Check sheet for the modelled part. Datum: model origin and axes. Units: mm. Face numbers are marked on the shaded views. Round coordinates to 2 decimals unless told otherwise and drop trailing zeros. Write each loop counter-clockwise with the first axis right and the second up, starting at its lowest first coordinate (ties: lowest second). Pieces come first, ordered by that corner, then holes.
Item 1: Cross-section at C-C on x = 91. Enter the section's corners in (y, z).
Item 2: Cross-section at A-A on z = 7.5. Enter the section's corners in (x, y), plus the area to 3 significant figures.
Item 3: Release check for a two-part mould opening along X. For the marked faces 1 and 2 record: +X half, -X half, draft (parallel to the pull), parting line (faces both ways), or undercut.
Item 4: Go/stop test with a flat-tipped pin: pin 1 Ø12 at (x, y) = (-1, -36.5) entering from +Z. Record where the tip stops, or that it passes through.
Item 5: Cross-section at B-B on y = -47. Enter the section's corners in (x, z), plus the area to 3 significant figures.
Item 6: Material ranges on line 1 (Y direction, x = -103.75, z = 1.75); line 2 (Y direction, x = 1.5, z = 7.5); line 3 (X direction, y = -32.5, z = 6.5), recorded low to high.
from build123d import *

# Parameters (mm, degrees)
PAD_DEPTH                     = 10
THICKNESS_T                   = -4
PAD001_DEPTH                  = 6
PAD001_MIRRORED_2_DEPTH       = 6
SKETCH003_R                   = 2
POCKET_DEPTH                  = 527.71231
SKETCH003_MIRRORED002_2_R     = 2
POCKET_MIRRORED002_2_DEPTH    = 527.71231
SKETCH004_R                   = 2.5
POCKET001_DEPTH               = 3
SKETCH004_MIRRORED004_2_R     = 2.5
POCKET001_MIRRORED004_2_DEPTH = 3


with BuildPart() as part:
    # Sketch → Pad (new body)
    with BuildSketch(Plane.XY):
        with BuildLine():
            Line((-103.75, -70), (103.75, -70))
            ThreePointArc((103.75, -70), (107.285534, -68.535534), (108.75, -65))
            Line((108.75, -65), (108.75, 65))
            ThreePointArc((108.75, 65), (107.285534, 68.535534), (103.75, 70))
            Line((103.75, 70), (-103.75, 70))
            ThreePointArc((-103.75, 70), (-107.285534, 68.535534), (-108.75, 65))
            Line((-108.75, 65), (-108.75, -65))
            ThreePointArc((-108.75, -65), (-107.285534, -68.535534), (-103.75, -70))
        make_face()
    extrude(amount=PAD_DEPTH)

    # Thickness
    thickness_openings = [part.faces().sort_by_distance(p)[0] for p in [
        (0, 0, 10),
    ]]
    offset(amount=THICKNESS_T, openings=thickness_openings)

    # Sketch002 (on Face10 of Thickness) → Pad001 (join)
    with BuildSketch(Plane.XY.offset(10)):
        with BuildLine():
            ThreePointArc((104.75, -58.071797), (98.800253, -60.050253), (96.821797, -66))
            Line((103.75, -66), (96.821797, -66))
            ThreePointArc((103.75, -66), (104.457107, -65.707107), (104.75, -65))
            Line((104.75, -65), (104.75, -58.071797))
        make_face()
    pad001 = extrude(amount=-PAD001_DEPTH)

    # Sketch002 Mirrored 2 → Pad001 Mirrored 2 (add)
    with BuildSketch(Plane(origin=(0, 0, 10), x_dir=(-1, 0, 0), z_dir=(0, 0, -1))):
        with BuildLine():
            ThreePointArc((104.75, -58.071797), (98.800253, -60.050253), (96.821797, -66))
            Line((103.75, -66), (96.821797, -66))
            ThreePointArc((103.75, -66), (104.457107, -65.707107), (104.75, -65))
            Line((104.75, -65), (104.75, -58.071797))
        make_face()
    pad001_mirrored_2 = extrude(amount=PAD001_MIRRORED_2_DEPTH)

    # Mirrored001: Pad001, Pad001 Mirrored 2 across XZ
    add(pad001.mirror(Plane.XZ))
    add(pad001_mirrored_2.mirror(Plane.XZ))

    # Sketch003 (on Face10 of MultiTransform) → Pocket (cut, through all)
    with BuildSketch(Plane.XY.offset(10)):
        with Locations((103.75, -65)):
            Circle(SKETCH003_R)
    pocket = extrude(amount=-POCKET_DEPTH, mode=Mode.SUBTRACT)

    # Sketch003 Mirrored002 2 → Pocket Mirrored002 2 (cut, through all)
    with BuildSketch(Plane(origin=(0, 0, 10), x_dir=(-1, 0, 0), z_dir=(0, 0, -1))):
        with Locations((103.75, -65)):
            Circle(SKETCH003_MIRRORED002_2_R)
    pocket_mirrored002_2 = extrude(amount=POCKET_MIRRORED002_2_DEPTH, mode=Mode.SUBTRACT)

    # Mirrored003: Pocket, Pocket Mirrored002 2 across XZ
    add(pocket.mirror(Plane.XZ), mode=Mode.SUBTRACT)
    add(pocket_mirrored002_2.mirror(Plane.XZ), mode=Mode.SUBTRACT)

    # Sketch004 (on Face4 of MultiTransform001) → Pocket001 (cut)
    with BuildSketch(Plane(origin=(0, 0, 0), x_dir=(1, 0, 0), z_dir=(0, 0, -1))):
        with Locations((103.75, -65)):
            Circle(SKETCH004_R)
    pocket001 = extrude(amount=-POCKET001_DEPTH, mode=Mode.SUBTRACT)

    # Sketch004 Mirrored004 2 → Pocket001 Mirrored004 2 (cut)
    with BuildSketch(Plane(origin=(0, 0, 0), x_dir=(-1, 0, 0), z_dir=(0, 0, 1))):
        with Locations((103.75, -65)):
            Circle(SKETCH004_MIRRORED004_2_R)
    pocket001_mirrored004_2 = extrude(amount=POCKET001_MIRRORED004_2_DEPTH, mode=Mode.SUBTRACT)

    # Mirrored005: Pocket001, Pocket001 Mirrored004 2 across XZ
    add(pocket001.mirror(Plane.XZ), mode=Mode.SUBTRACT)
    add(pocket001_mirrored004_2.mirror(Plane.XZ), mode=Mode.SUBTRACT)


solid = part.part
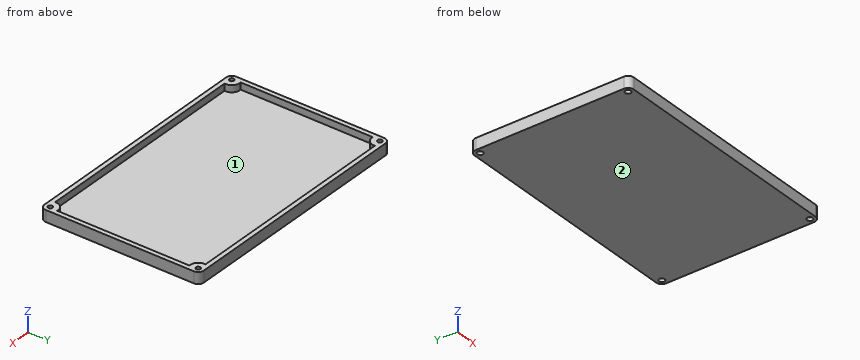
Response values:
1. outline: (-70, 0) - (70, 0) - (70, 10) - (66, 10) - (66, 4) - (-66, 4) - (-66, 10) - (-70, 10) - close
2. outline: (-108.75, -65) arc R5 ccw to (-103.75, -70) - (103.75, -70) arc R5 ccw to (108.75, -65) - (108.75, 65) arc R5 ccw to (103.75, 70) - (-103.75, 70) arc R5 ccw to (-108.75, 65) - close; hole circle Ø4 at (-103.75, -65); hole circle Ø4 at (-103.75, 65); hole (-104.75, -58.07) arc R7 cw to (-96.82, -66) - (96.82, -66) arc R7 cw to (104.75, -58.07) - (104.75, 58.07) arc R7 cw to (96.82, 66) - (-96.82, 66) arc R7 cw to (-104.75, 58.07) - close; hole circle Ø4 at (103.75, -65); hole circle Ø4 at (103.75, 65)
2. area: 2,940 mm2
3. face 1: undercut
3. face 2: draft
4. pin 1: stops at z = 4
5. outline: (-108.75, 0) - (108.75, 0) - (108.75, 10) - (104.75, 10) - (104.75, 4) - (-104.75, 4) - (-104.75, 10) - (-108.75, 10) - close
5. area: 918 mm2
6. line 1: y = -70 to -67.5, -62.5 to 62.5, 67.5 to 70
6. line 2: y = -70 to -66, 66 to 70
6. line 3: x = -108.75 to -104.75, 104.75 to 108.75
